Could you check a few things on this model? Use its own coordinates, in mm. Face numbers are marked on the shaded views. A direction names the side the tool comes from. Round coordinates to 2 decimals unless told otherwise and drop trailing zeros. Loops run counter-clockwise (first coordinate to the right, second up) from the corner with the lowest first, then second, coordinate; pieces in that order, holes last. Notation, with made-up numbers: M 85,6.5 L 120,6.5 A25 cw 120,34.5 Z; hole C -34.75,72 d9. An arc over 180 degrees is marked long. Answer in a Markdown table with one row per item.
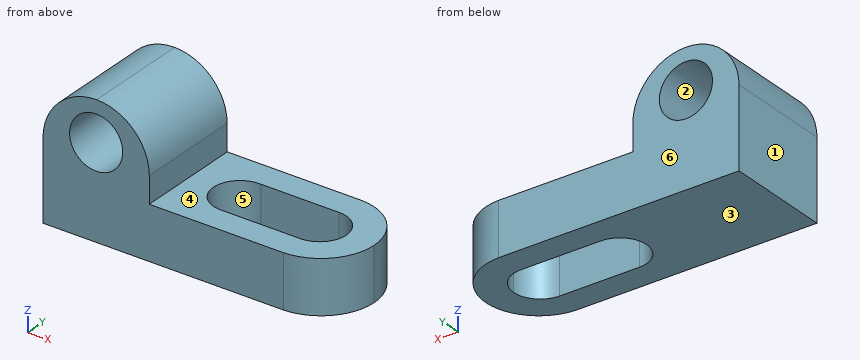
```python
from build123d import *

# Parameters (mm, degrees)
F1_DEPTH = 25.4
F2_R     = 6.35
F3_DEPTH = 25.401
F5_DEPTH = 25.4
F7_DEPTH = 12.701
F9_DEPTH = 12.701


# Not quite as in the source:
# - ends of sketch curves that miss each other by under 0.0002 mm in the source are joined


with BuildPart() as f1:
    # F0 (on Front) → F1 (new body)
    with BuildSketch(Plane.XZ):
        Polygon((-31.4219513942, 31.5156808858), (-56.8219513942, 31.75), (-56.8219513942, 0), (13.0280486058, 0), (13.0280486058, 12.7), (-31.4219513942, 12.7), align=None)
    extrude(amount=F1_DEPTH)

    # F2 (on face) → F3 (cut, through all)
    with BuildSketch(Plane.XZ.offset(25.4)):
        with Locations((-44.1219513942, 22.1078404429)):
            Circle(F2_R)
    extrude(amount=-F3_DEPTH, mode=Mode.SUBTRACT)

    # F4 (on face) → F5 (cut)
    with BuildSketch(Plane.XZ.offset(25.4)):
        with BuildLine():
            ThreePointArc((-56.8219513942, 19.05), (-53.0189875224, 27.9952387553), (-44.0048017085, 31.6317597181))
            Line((-44.0048017085, 31.6317597181), (-56.8219513942, 31.75))
            Line((-56.8219513942, 31.75), (-56.8219513942, 19.05))
        make_face()
        with BuildLine():
            ThreePointArc((-44.0048017085, 31.6317597181), (-35.1409409401, 27.9120157755), (-31.4219513942, 19.0478384602))
            Line((-31.4219513942, 19.0478384602), (-31.4219513942, 31.5156808858))
            Line((-31.4219513942, 31.5156808858), (-44.0048017085, 31.6317597181))
        make_face()
    extrude(amount=-F5_DEPTH, mode=Mode.SUBTRACT)

    # F6 (on face) → F7 (cut, through all)
    with BuildSketch(Plane.XY.offset(12.7)):
        with BuildLine():
            ThreePointArc((-19.05, -19.05), (-14.5598719395, -17.1901280605), (-12.7, -12.7))
            ThreePointArc((-12.7, -12.7), (-14.4299815751, -8.3436334229), (-18.6773007098, -6.3609468184))
            ThreePointArc((-18.6773007098, -6.3609468184), (-25.3972627054, -12.5135699905), (-19.05, -19.05))
        make_face()
        with BuildLine():
            ThreePointArc((-18.6773007098, -6.3609468184), (-14.4299815751, -8.3436334229), (-12.7, -12.7))
            ThreePointArc((-12.7, -12.7), (-14.5598719395, -17.1901280605), (-19.05, -19.05))
            Line((-19.05, -19.05), (0, -19.05))
            ThreePointArc((0, -19.05), (4.4901280605, -17.1901280605), (6.35, -12.7))
            ThreePointArc((6.35, -12.7), (4.4901280605, -8.2098719395), (0, -6.35))
            Line((0, -6.35), (-18.6773007098, -6.3609468184))
        make_face()
    extrude(amount=-F7_DEPTH, mode=Mode.SUBTRACT)

    # F8 (on face) → F9 (cut, through all)
    with BuildSketch(Plane.XY.offset(12.7)):
        with BuildLine():
            ThreePointArc((0.6478368888, 0), (9.420896658, -3.8320853331), (13.0280486058, -12.7))
            Line((13.0280486058, -12.7), (13.0280486058, 0))
            Line((13.0280486058, 0), (0.6478368888, 0))
        make_face()
        with BuildLine():
            ThreePointArc((13.0280486058, -12.7), (9.420896658, -21.5679146669), (0.6478368888, -25.4))
            Line((0.6478368888, -25.4), (13.0280486058, -25.4))
            Line((13.0280486058, -25.4), (13.0280486058, -12.7))
        make_face()
    extrude(amount=-F9_DEPTH, mode=Mode.SUBTRACT)


solid = f1.part
```
1) I want a section at A-A, the plane y = -12. Please give me the cut outline in (x, z).
Computed:
| item | result |
|---|---|
| outline | M -56.82,0 L -25.36,0 L -25.36,12.7 L -31.42,12.7 L -31.42,19.05 A12.7 ccw -56.82,19.05 Z; M 6.31,0 L 13.01,0 L 13.01,12.7 L 6.31,12.7 Z; hole C -44.12,22.11 d12.7 |
2) I want a section at D-D, the plane y = -20. Please give me the cut outline in (x, z), plus the area to 3 significant figures.
Computed:
| item | result |
|---|---|
| outline | M -56.82,0 L 10.72,0 L 10.72,12.7 L -31.42,12.7 L -31.42,19.05 A12.7 ccw -56.82,19.05 Z; hole C -44.12,22.11 d12.7 |
| area | 1,140 mm² |
3) Will these pins go through, and if not, where does the flat tip stop? P1, Ø3, axis at y = -8, z = 16, coming from the +X side; P2, Ø6, axis at x = -25.5, y = -5, coming from the +Z side; P3, Ø3, axis at y = -20, z = 25, coming from the +X side.
Computed:
| item | result |
|---|---|
| P1 | stops at x = -31.42 |
| P2 | stops at z = 12.7 |
| P3 | stops at x = -32.27 |
4) I want a section at C-C, the plane x = -48.5. Please give me the cut outline in (y, z), plus the area to 3 significant figures.
Computed:
| item | result |
|---|---|
| outline | M -25.4,0 L 0,0 L 0,17.51 L -25.4,17.51 Z; M -25.4,26.71 L 0,26.71 L 0,30.85 L -25.4,30.85 Z |
| area | 550 mm² |
5) Which directions (+Z, -Z, +X, -X, +Y, -Y) give clear straight access to the entire face, cutting with the end or side of a thin tool? Please do the marked faces 4, 5 and 6.
Computed:
| item | result |
|---|---|
| face 4 | +Z, +X, +Y, -Y |
| face 5 | +Z, -Z |
| face 6 | +Z, -Z, +X, -X, +Y |
6) If we mould it in two halves opening along X, with no side actions, what happens to the marked faces 1, 2 and 3? For each: released by +X, released by -X, zero draft, split by the parting line, or undercut.
Computed:
| item | result |
|---|---|
| face 1 | released by -X |
| face 2 | undercut |
| face 3 | zero draft |
7) I need wall thicknesses on line 1 (Y direction, x = -15.5, z = 5.5); line 2 (Z direction, x = 3.5, y = -3); line 3 (X direction, y = -10.5, z = 7). Which ranges of each line are inside material? Lowest first, please.
Computed:
| item | result |
|---|---|
| line 1 | y = -25.4 to -19.05, -6.36 to 0 |
| line 2 | z = 0 to 12.7 |
| line 3 | x = -56.82 to -25.01, 5.96 to 12.84 |
